from build123d import *

# Parameters (mm, degrees)
F0_R     = 2.5
F1_DEPTH = 2
F2_R     = 2
F0_R_2   = 1.4
F3_DEPTH = 3


with BuildPart() as f1:
    # F0 (on Top) → F1 (new body)
    with BuildSketch(Plane.XY):
        Polygon((-35, -5), (35, -5), (35, 5), (0, 5), (-35, 5), (-35, 3.662193), align=None)
        Circle(F0_R, mode=Mode.SUBTRACT)
    extrude(amount=F1_DEPTH)

    # F2
    f2_edges = [f1.edges().sort_by_distance(p)[0] for p in [
        (-35, 5, 1),
        (-35, -5, 1),
        (35, -5, 1),
        (35, 5, 1),
    ]]
    fillet(f2_edges, radius=F2_R)

    # F0 (on Top) → F3 (join)
    with BuildSketch(Plane.XY):
        Circle(F0_R)
        Circle(F0_R_2, mode=Mode.SUBTRACT)
    extrude(amount=F3_DEPTH)


solid = f1.part
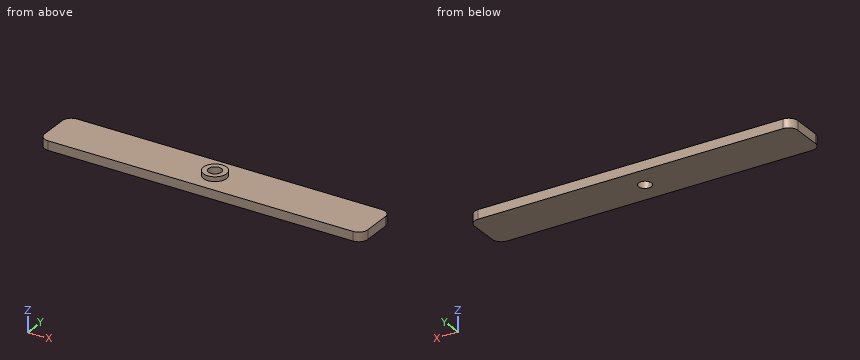
Design review of the part built by this model. Coordinates are the model's own, in mm. Give positions to 0.01 mm unless a question says otherwise; leave off trailing zeros. Loops run counter-clockwise (first coordinate to the right, second up) from the corner with the lowest first, then second, coordinate; pieces in that order, holes last. Notation, with made-up numbers: M -8.75,66 L 4.25,66 A21 cw 4.25,104 Z; hole C 68,-30.5 d4. An arc over 180 degrees is marked long. One line per question, with ' | ' between items. Start each with the question number.
1. Add section D-D (x = 28.5). Write out the cut boundary in (y, z), plus the area to 3 significant figures.
2. To check wall thickness, follow L1, parallel to Y at x = 0, z = 1.4; L2, parallel to Z at x = 0, y = 4; L3, parallel to X at y = -0.5, z = 0.3. State the ranges of each line that lie inside material, in increasing order.
3. Add section A-A (y = 0). Write out the cut boundary in (x, z).
4. Insertion check: P1, Ø4.5, axis at x = 0, y = 0, coming from the -Z side. The pin has a flat end and moves straight along its axis. Give the tip position at first contact, or say it passes through.
5. Add section C-C (z = 2.45). Write out the cut boundary in (x, y), plus the area to 3 significant figures.
6. Add section B-B (x = 0). Write out the cut boundary in (y, z).
Worked out:
1) outline: M -5,0 L 5,0 L 5,2 L -5,2 Z | area: 20.0 mm²
2) L1: y = -5 to -1.4, 1.4 to 5 | L2: z = 0 to 2 | L3: x = -35 to -1.31, 1.31 to 35
3) outline: M -35,0 L -1.4,0 L -1.4,3 L -2.5,3 L -2.5,2 L -35,2 Z; M 1.4,0 L 35,0 L 35,2 L 2.5,2 L 2.5,3 L 1.4,3 Z
4) P1: stops at z = 0
5) outline: C 0,0 d5; hole C 0,0 d2.8 | area: 13.5 mm²
6) outline: M -5,0 L -1.4,0 L -1.4,3 L -2.5,3 L -2.5,2 L -5,2 Z; M 1.4,0 L 5,0 L 5,2 L 2.5,2 L 2.5,3 L 1.4,3 Z
